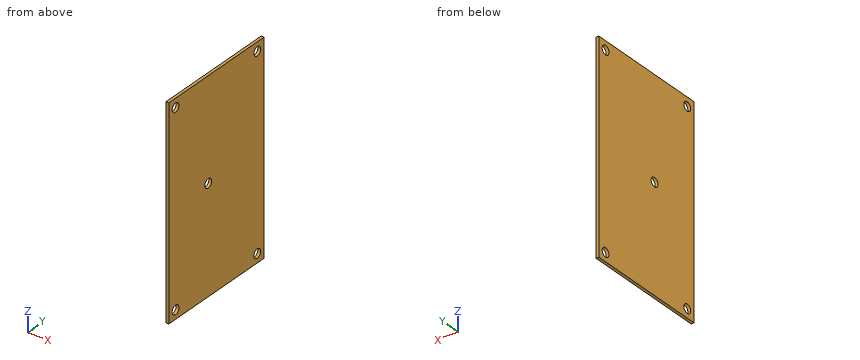
```python
from build123d import *

# Parameters (mm, degrees)
SKETCH1_W           = 117
SKETCH1_H           = 70
BOSS_EXTRUDE1_DEPTH = 1.6
SKETCH2_R           = 2.5
CUT_EXTRUDE1_DEPTH  = 2.6


with BuildPart() as part:
    # Sketch1 → Boss-Extrude1 (new body)
    with BuildSketch(Plane(origin=(0, 0, 0), x_dir=(0, 0, -1), z_dir=(1, 0, 0))):
        with Locations((58.5, 35)):
            Rectangle(SKETCH1_W, SKETCH1_H)
    extrude(amount=BOSS_EXTRUDE1_DEPTH)

    # Sketch2 → Cut-Extrude1 (cut, through all)
    with BuildSketch(Plane(origin=(1.6, 0, 0), x_dir=(0, 0, -1), z_dir=(1, 0, 0))):
        with Locations((5, 65)):
            Circle(SKETCH2_R)
        with Locations((5, 5)):
            Circle(SKETCH2_R)
        with Locations((112, 5)):
            Circle(SKETCH2_R)
        with Locations((112, 65)):
            Circle(SKETCH2_R)
        with Locations((57, 29)):
            Circle(SKETCH2_R)
    extrude(amount=-CUT_EXTRUDE1_DEPTH, mode=Mode.SUBTRACT)


solid = part.part
```
CAD build for the part. Positions are in the model's coordinates, mm. Round coordinates to 2 decimals unless told otherwise and drop trailing zeros. Write each loop counter-clockwise with the first axis right and the second up, starting at its lowest first coordinate (ties: lowest second). Pieces come first, ordered by that corner, then holes. Notation, with made-up numbers: (71, 38.25) - (112, 38.25) arc R31 cw to (112, 64.25) - close; hole circle Ø9 at (66.25, -10). An arc over 180 degrees is marked (long way). Return JSON: item names as keys, results as strings. Group by question number.
Item 1: Band-saw the part on A-A on z = -112. List the corners of the cut face in (x, y).
Item 2: Probe probe 1 along Y at (x, z) = (1.2, -112); probe 2 along Y at (x, z) = (0.9, -5.5); probe 3 along Y at (x, z) = (0.55, -59). List the from-to ranges inside material, lowest first.
Item 3: Band-saw the part on B-B on y = 29. List the corners of the cut face in (x, z), plus the area to 3 significant figures.
Resolved:
{
 "1": {"outline": "(0, 0) - (1.6, 0) - (1.6, 2.5) - (0, 2.5) - close; (0, 7.5) - (1.6, 7.5) - (1.6, 62.5) - (0, 62.5) - close; (0, 67.5) - (1.6, 67.5) - (1.6, 70) - (0, 70) - close"},
 "2": {"probe 1": "y = 0 to 2.5, 7.5 to 62.5, 67.5 to 70", "probe 2": "y = 0 to 2.55, 7.45 to 62.55, 67.45 to 70", "probe 3": "y = 0 to 27.5, 30.5 to 70"},
 "3": {"outline": "(0, -117) - (1.6, -117) - (1.6, -59.5) - (0, -59.5) - close; (0, -54.5) - (1.6, -54.5) - (1.6, 0) - (0, 0) - close", "area": "179 mm²"}
}
